Part model, mm, in its own coordinate system. Give positions to 0.01 mm unless a question says otherwise; leave off trailing zeros. Loops run counter-clockwise (first coordinate to the right, second up) from the corner with the lowest first, then second, coordinate; pieces in that order, holes last. Notation, with made-up numbers: M 20,36.25 L 72,36.25 A6 cw 72,45.25 Z; hole C 76.25,60.25 d8. An arc over 180 degrees is marked long. Answer in a Markdown table with one row per item.
from build123d import *

# Parameters (mm, degrees)
F0_W     = 270
F0_H     = 200
F1_DEPTH = 3
F2_W     = 30.5
F2_H     = 3.5
F2_W_2   = 3.5
F2_H_2   = 30.5
F2_H_3   = 29
F3_DEPTH = 3


with BuildPart() as f1:
    # F0 (on Top) → F1 (new body)
    with BuildSketch(Plane.XY):
        Rectangle(F0_W, F0_H)
    extrude(amount=F1_DEPTH)

    # F2 (on face) → F3 (cut)
    with BuildSketch(Plane.XY.offset(3)):
        with Locations((84.75, 88.25)):
            Rectangle(F2_W, F2_H)
        with Locations((29.25, 88.25)):
            Rectangle(F2_W, F2_H)
        with Locations((123.25, 49.75)):
            Rectangle(F2_W_2, F2_H_2)
        with Locations((-84.75, 88.25)):
            Rectangle(F2_W, F2_H)
        with Locations((-29.25, 88.25)):
            Rectangle(F2_W, F2_H)
        Polygon((-84.75, -88.25), (-100, -90), (-84.75, -90), align=None)
        Polygon((-100, -86.5), (-100, -90), (-84.75, -88.25), align=None)
        Polygon((-69.5, -86.5), (-100, -86.5), (-84.75, -88.25), align=None)
        Polygon((-84.75, -88.25), (-84.75, -90), (-69.5, -90), align=None)
        Polygon((-69.5, -86.5), (-84.75, -88.25), (-69.5, -90), align=None)
        with Locations((29.25, -88.25)):
            Rectangle(F2_W, F2_H)
        Polygon((-29.25, -88.25), (-44.5, -90), (-29.25, -90), align=None)
        Polygon((-44.5, -86.5), (-44.5, -90), (-29.25, -88.25), align=None)
        Polygon((-14, -86.5), (-44.5, -86.5), (-29.25, -88.25), align=None)
        Polygon((-29.25, -88.25), (-29.25, -90), (-14, -90), align=None)
        Polygon((-14, -86.5), (-29.25, -88.25), (-14, -90), align=None)
        with Locations((84.75, -88.25)):
            Rectangle(F2_W, F2_H)
        with Locations((123.25, -49.75)):
            Rectangle(F2_W_2, F2_H_2)
        with Locations((-123.25, -49.75)):
            Rectangle(F2_W_2, F2_H_2)
        with Locations((-123.25, 49.75)):
            Rectangle(F2_W_2, F2_H_2)
        with Locations((123.25, 0)):
            Rectangle(F2_W_2, F2_H_3)
        with Locations((-123.25, 0)):
            Rectangle(F2_W_2, F2_H_3)
    extrude(amount=-F3_DEPTH, mode=Mode.SUBTRACT)


solid = f1.part
(1) Drill centre lines: line 1 along X through (y, z) = (-10, 0.75); line 2 along Y through (x, z) = (70, 2.05); line 3 along Y through (x, z) = (-124, 1.95). Where is each one in solid material? Low to high.
Recorded:
| item | result |
|---|---|
| line 1 | x = -135 to -125, -121.5 to 121.5, 125 to 135 |
| line 2 | y = -100 to -90, -86.5 to 86.5, 90 to 100 |
| line 3 | y = -100 to -65, -34.5 to -14.5, 14.5 to 34.5, 65 to 100 |
(2) Saw through at A-A (x = 37). Write the cut outline in (y, z).
Recorded:
| item | result |
|---|---|
| outline | M -100,0 L -90,0 L -90,3 L -100,3 Z; M -86.5,0 L 86.5,0 L 86.5,3 L -86.5,3 Z; M 90,0 L 100,0 L 100,3 L 90,3 Z |
(3) Saw through at C-C (z = 0.8). Give the number of separate pieces and of enclosed holes in the cut face, plus the area to 3 significant figures.
Recorded:
| item | result |
|---|---|
| separate pieces | 1 |
| enclosed holes | 14 |
| area | 52,500 mm^2 |
(4) Saw through at B-B (y = 59). Write the cut outline in (x, z).
Recorded:
| item | result |
|---|---|
| outline | M -135,0 L -125,0 L -125,3 L -135,3 Z; M -121.5,0 L 121.5,0 L 121.5,3 L -121.5,3 Z; M 125,0 L 135,0 L 135,3 L 125,3 Z |
(5) Pin check, flat tip, straight feed: pin 1 Ø8 at (x, y) = (93, 74) entering from -Z. Stop position of the tip, or through.
Recorded:
| item | result |
|---|---|
| pin 1 | stops at z = 0 |
